from build123d import *

# Parameters (mm, degrees)
EXTRUDE_1_DEPTH        = 4
HOLE_WIZARD_M3_1_D     = 3
HOLE_WIZARD_M3_1_DEPTH = 10
HOLE_WIZARD_M3_1_TIP   = 0.901290929


with BuildPart() as part:
    # 草图1 → 凸台-拉伸1 (new body)
    with BuildSketch(Plane.XY):
        with BuildLine():
            Line((7.985331622, 162.373829532), (7.985331622, 17.626170468))
            Line((7.985331622, 17.626170468), (9.80962292, 19.515279408))
            ThreePointArc((9.80962292, 19.515279408), (16.920274479, 21.026695055), (20.985331622, 15))
            Line((20.985331622, 15), (20.985331622, 165))
            ThreePointArc((20.985331622, 165), (16.920274479, 158.973304945), (9.80962292, 160.484720592))
            Line((9.80962292, 160.484720592), (7.985331622, 162.373829532))
        make_face()
        with BuildLine():
            Line((-4.675708702, 175.484720592), (7.985331622, 162.373829532))
            Line((7.985331622, 162.373829532), (7.985331622, 165))
            ThreePointArc((7.985331622, 165), (12.050388765, 171.026695055), (19.161040324, 169.515279408))
            Line((19.161040324, 169.515279408), (4.675708702, 184.515279408))
            ThreePointArc((4.675708702, 184.515279408), (-4.515279408, 184.675708702), (-4.675708702, 175.484720592))
        make_face()
        with BuildLine():
            Line((7.985331622, 165), (7.985331622, 162.373829532))
            Line((7.985331622, 162.373829532), (9.80962292, 160.484720592))
            ThreePointArc((9.80962292, 160.484720592), (16.920274479, 158.973304945), (20.985331622, 165))
            ThreePointArc((20.985331622, 165), (20.512026677, 167.434942857), (19.161040324, 169.515279408))
            ThreePointArc((19.161040324, 169.515279408), (12.050388765, 171.026695055), (7.985331622, 165))
        make_face()
        with BuildLine():
            Line((9.80962292, 19.515279408), (7.985331622, 17.626170468))
            Line((7.985331622, 17.626170468), (7.985331622, 15))
            ThreePointArc((7.985331622, 15), (12.050388765, 8.973304945), (19.161040324, 10.484720592))
            ThreePointArc((19.161040324, 10.484720592), (20.512026677, 12.565057143), (20.985331622, 15))
            ThreePointArc((20.985331622, 15), (16.920274479, 21.026695055), (9.80962292, 19.515279408))
        make_face()
        with BuildLine():
            Line((7.985331622, 17.626170468), (-4.675708702, 4.515279408))
            ThreePointArc((-4.675708702, 4.515279408), (-4.515279408, -4.675708702), (4.675708702, -4.515279408))
            Line((4.675708702, -4.515279408), (19.161040324, 10.484720592))
            ThreePointArc((19.161040324, 10.484720592), (12.050388765, 8.973304945), (7.985331622, 15))
            Line((7.985331622, 15), (7.985331622, 17.626170468))
        make_face()
    extrude(amount=EXTRUDE_1_DEPTH)

    # M3 螺纹孔1
    with Locations(Plane.XY.offset(4)):
        with Locations((0, 0), (0, 180)):
            Hole(HOLE_WIZARD_M3_1_D / 2, depth=HOLE_WIZARD_M3_1_DEPTH)
            with Locations((0, 0, -(HOLE_WIZARD_M3_1_DEPTH + HOLE_WIZARD_M3_1_TIP / 2))):  # 118° drill point
                Cone(0, HOLE_WIZARD_M3_1_D / 2, HOLE_WIZARD_M3_1_TIP, mode=Mode.SUBTRACT)


solid = part.part
CAD build for the part. Positions are in the model's coordinates, mm. A direction names the side the tool comes from. Round coordinates to 2 decimals unless told otherwise and drop trailing zeros. Order: outer loops, then holes, each group sorted by start corner. A loop starts at its lowest first (then second) coordinate and runs counter-clockwise, first axis right, second up. Notation, with made-up numbers: (84, 15.25) -> (110, 15.25) arc R10 cw to (110, 32.25) -> close; hole circle Ø7 at (-16.75, 78). An arc over 180 degrees is marked (long way). Write each question's results on one line, items separated by ' | '.
1. Cut at A-A (z = 1.2). Give the cut face in (x, y), plus the area to 3 significant figures.
Findings below:
outline: (-4.68, 4.52) arc R6.5 ccw to (4.68, -4.52) -> (19.16, 10.48) arc R6.5 ccw to (20.99, 15) -> (20.99, 165) arc R6.5 ccw to (19.16, 169.52) -> (4.68, 184.52) arc R6.5 ccw to (-4.68, 175.48) -> (7.99, 162.37) -> (7.99, 17.63) -> close; hole circle Ø3 at (0, 0); hole circle Ø3 at (0, 180) | area: 2,610 mm²
2. Pull direction Y, two halves, no side cores. Call faces 3 (the face through (10, 91, 4)), 4 (the face through (12.02, 176.91, 1.97)), 5 (the face through (1.566, 169.021, 1.972)), 6 (the face through (11.82, 2.88, 1.97)): pulls with the +Y half, pulls with the -Y half, needs draft (parallel to the pull), parting line crosses it, or undercut.
Findings below:
face 3: needs draft | face 4: pulls with the +Y half | face 5: undercut | face 6: pulls with the -Y half
3. 3-axis set-ups, long thin cutter, end or side, ignore diameter. For faces 1 (the face through (0.195, 181.487, 1.972)), 2 (the face through (1.74, 11.16, 1.97)): which of +Z, -Z, +X, -X, +Y, -Y reach the whole face in a straight line?
Findings below:
face 1: +Z, -Z | face 2: +Z, -Z, -X
4. Cut at B-B (y = 104.5). Give the cut face in (x, z).
Findings below:
outline: (7.99, 0) -> (20.99, 0) -> (20.99, 4) -> (7.99, 4) -> close
5. Wall check: line 1 along Y through (x, z) = (0, 2.9); line 2 along Y through (x, z) = (-0.75, 1.45); line 3 along X through (y, z) = (129, 1.9). Give the ranges that are in metal, low to high. Write a range as [from, to].
Findings below:
line 1: y = [-6.5, -1.5], [1.5, 9.36], [170.64, 178.5], [181.5, 186.5] | line 2: y = [-6.46, -1.3], [1.3, 8.58], [171.42, 178.7], [181.3, 186.46] | line 3: x = [7.99, 20.99]
6. Cut at C-C (y = 172). Give the cut face in (x, z), plus the area to 3 significant figures.
Findings below:
outline: (-1.31, 0) -> (16.76, 0) -> (16.76, 4) -> (-1.31, 4) -> close | area: 72.3 mm²
7. Flat gauge pin, fed straight in: P1, Ø1, axis at x = 5, z = 3, coming from the -Y side. Where does the tip first touch, or does it go through?
Findings below:
P1: stops at y = -4.69
